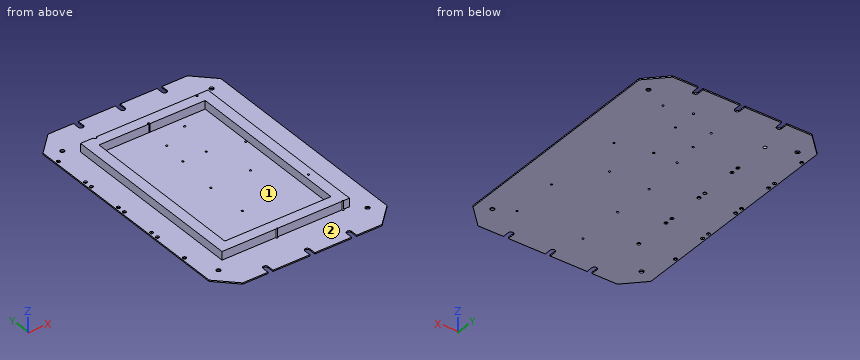
from build123d import *

# Parameters (mm, degrees)
BOSS_EXTRUDE1_DEPTH      = 0.75
BOSS_EXTRUDE1_DEPTH_BACK = 0.75
CUT_EXTRUDE1_DEPTH       = 190.772483022
LPATTERN1_COUNT          = 7
LPATTERN1_PITCH          = 50
MIRROR1_COPY_1_DEPTH     = 190.772483022
MIRROR1_COPY_2_DEPTH     = 190.772483022
MIRROR1_COPY_3_DEPTH     = 190.772483022
MIRROR1_COPY_4_DEPTH     = 190.772483022
MIRROR1_COPY_5_DEPTH     = 190.772483022
MIRROR1_COPY_6_DEPTH     = 190.772483022
SKETCH6_W                = 152.4
SKETCH6_H                = 228.6
SKETCH6_W_2              = 127
SKETCH6_H_2              = 203.2
BOSS_EXTRUDE2_DEPTH      = 11.5
SKETCH7_R                = 2.54
CUT_EXTRUDE2_DEPTH       = 191.11912795
CUT_EXTRUDE3_DEPTH       = 191.11912795
CUT_EXTRUDE3_DEPTH_BACK  = 191.11912795
SKETCH8_R                = 1.15
CUT_EXTRUDE4_DEPTH       = 191.11912795


with BuildPart() as part:
    # Sketch3 → Boss-Extrude1 (new, two sides: drawn at the far end of the back side and taken through both)
    with BuildSketch(Plane.XY.offset(-BOSS_EXTRUDE1_DEPTH_BACK)):
        Polygon((-106.3625, 134.1625), (-83.3625, 157.1625), (83.3625, 157.1625), (106.3625, 134.1625), (106.3625, -134.1625), (83.3625, -157.1625), (-83.3625, -157.1625), (-106.3625, -134.1625), align=None)
    extrude(amount=BOSS_EXTRUDE1_DEPTH + BOSS_EXTRUDE1_DEPTH_BACK)

    # Sketch4 → Cut-Extrude1 (cut, symmetric)
    with BuildSketch(Plane.XY):
        with BuildLine():
            Line((53, 149.225), (53, 157.1625))
            Line((53, 157.1625), (47, 157.1625))
            Line((47, 157.1625), (47, 149.225))
            ThreePointArc((47, 149.225), (50, 146.225), (53, 149.225))
        make_face()
    cut_extrude1 = extrude(amount=CUT_EXTRUDE1_DEPTH, both=True, mode=Mode.SUBTRACT)

    # LPattern1: Cut-Extrude1 ×7
    with Locations(*[(-i * LPATTERN1_PITCH, 0, 0) for i in range(1, LPATTERN1_COUNT)]):
        add(cut_extrude1, mode=Mode.SUBTRACT)

    # Mirror1: Cut-Extrude1 across plane
    add(cut_extrude1.mirror(Plane.ZX), mode=Mode.SUBTRACT)

    # Mirror1 copy 1 sketch → Mirror1 copy 1 (cut, symmetric)
    with BuildSketch(Plane(origin=(-50, 0, 0), x_dir=(1, 0, 0), z_dir=(0, 0, 1))):
        with BuildLine():
            Line((53, -149.225), (53, -157.1625))
            Line((53, -157.1625), (47, -157.1625))
            Line((47, -157.1625), (47, -149.225))
            ThreePointArc((47, -149.225), (50, -146.225), (53, -149.225))
        make_face()
    extrude(amount=MIRROR1_COPY_1_DEPTH, both=True, mode=Mode.SUBTRACT)

    # Mirror1 copy 2 sketch → Mirror1 copy 2 (cut, symmetric)
    with BuildSketch(Plane(origin=(-100, 0, 0), x_dir=(1, 0, 0), z_dir=(0, 0, 1))):
        with BuildLine():
            Line((53, -149.225), (53, -157.1625))
            Line((53, -157.1625), (47, -157.1625))
            Line((47, -157.1625), (47, -149.225))
            ThreePointArc((47, -149.225), (50, -146.225), (53, -149.225))
        make_face()
    extrude(amount=MIRROR1_COPY_2_DEPTH, both=True, mode=Mode.SUBTRACT)

    # Mirror1 copy 3 sketch → Mirror1 copy 3 (cut, symmetric)
    with BuildSketch(Plane(origin=(-150, 0, 0), x_dir=(1, 0, 0), z_dir=(0, 0, 1))):
        with BuildLine():
            Line((53, -149.225), (53, -157.1625))
            Line((53, -157.1625), (47, -157.1625))
            Line((47, -157.1625), (47, -149.225))
            ThreePointArc((47, -149.225), (50, -146.225), (53, -149.225))
        make_face()
    extrude(amount=MIRROR1_COPY_3_DEPTH, both=True, mode=Mode.SUBTRACT)

    # Mirror1 copy 4 sketch → Mirror1 copy 4 (cut, symmetric)
    with BuildSketch(Plane(origin=(-200, 0, 0), x_dir=(1, 0, 0), z_dir=(0, 0, 1))):
        with BuildLine():
            Line((53, -149.225), (53, -157.1625))
            Line((53, -157.1625), (47, -157.1625))
            Line((47, -157.1625), (47, -149.225))
            ThreePointArc((47, -149.225), (50, -146.225), (53, -149.225))
        make_face()
    extrude(amount=MIRROR1_COPY_4_DEPTH, both=True, mode=Mode.SUBTRACT)

    # Mirror1 copy 5 sketch → Mirror1 copy 5 (cut, symmetric)
    with BuildSketch(Plane(origin=(-250, 0, 0), x_dir=(1, 0, 0), z_dir=(0, 0, 1))):
        with BuildLine():
            Line((53, -149.225), (53, -157.1625))
            Line((53, -157.1625), (47, -157.1625))
            Line((47, -157.1625), (47, -149.225))
            ThreePointArc((47, -149.225), (50, -146.225), (53, -149.225))
        make_face()
    extrude(amount=MIRROR1_COPY_5_DEPTH, both=True, mode=Mode.SUBTRACT)

    # Mirror1 copy 6 sketch → Mirror1 copy 6 (cut, symmetric)
    with BuildSketch(Plane(origin=(-300, 0, 0), x_dir=(1, 0, 0), z_dir=(0, 0, 1))):
        with BuildLine():
            Line((53, -149.225), (53, -157.1625))
            Line((53, -157.1625), (47, -157.1625))
            Line((47, -157.1625), (47, -149.225))
            ThreePointArc((47, -149.225), (50, -146.225), (53, -149.225))
        make_face()
    extrude(amount=MIRROR1_COPY_6_DEPTH, both=True, mode=Mode.SUBTRACT)

    # Sketch6 → Boss-Extrude2 (add)
    with BuildSketch(Plane(origin=(0, 0, -0.75), x_dir=(-1, 0, 0), z_dir=(0, 0, -1))):
        Rectangle(SKETCH6_W, SKETCH6_H)
        Rectangle(SKETCH6_W_2, SKETCH6_H_2, mode=Mode.SUBTRACT)
    extrude(amount=-BOSS_EXTRUDE2_DEPTH)

    # Sketch7 → Cut-Extrude2 (cut, through all)
    with BuildSketch(Plane(origin=(0, 0, -0.75), x_dir=(-1, 0, 0), z_dir=(0, 0, -1))):
        with Locations((89.2175, 126.0475)):
            Circle(SKETCH7_R)
        with Locations((-89.2175, 126.0475)):
            Circle(SKETCH7_R)
        with Locations((-89.2175, -126.0475)):
            Circle(SKETCH7_R)
        with Locations((89.2175, -126.0475)):
            Circle(SKETCH7_R)
    extrude(amount=-CUT_EXTRUDE2_DEPTH, mode=Mode.SUBTRACT)

    # Sketch8 → Cut-Extrude3 (cut, two sides: drawn at the far end of the back side and taken through both)
    with BuildSketch(Plane(origin=(0, 0, -0.75), x_dir=(-1, 0, 0), z_dir=(0, 0, -1)).offset(-CUT_EXTRUDE3_DEPTH_BACK)):
        with Locations((-30.1625, 119.0625)):
            Circle(SKETCH8_R)
        with Locations((3.3375, 102.5625)):
            Circle(SKETCH8_R)
        with Locations((-30.1625, 89.8625)):
            Circle(SKETCH8_R)
        with Locations((3.3375, 73.3625)):
            Circle(SKETCH8_R)
        with Locations((-21.2725, 42.8625)):
            Circle(SKETCH8_R)
        with Locations((6.6675, 42.8625)):
            Circle(SKETCH8_R)
        with Locations((-36.5125, -7.9375)):
            Circle(SKETCH8_R)
        with Locations((11.7475, -9.2075)):
            Circle(SKETCH8_R)
        with Locations((-68.2625, -58.7375)):
            Circle(SKETCH8_R)
        with Locations((10.7375, -58.7375)):
            Circle(SKETCH8_R)
        with Locations((10.7375, -114.7375)):
            Circle(SKETCH8_R)
        with Locations((-68.2625, -114.7375)):
            Circle(SKETCH8_R)
        with Locations((-61.9125, 112.7125)):
            Circle(SKETCH8_R)
        with Locations((-61.9125, 33.7125)):
            Circle(SKETCH8_R)
    extrude(amount=CUT_EXTRUDE3_DEPTH + CUT_EXTRUDE3_DEPTH_BACK, mode=Mode.SUBTRACT)

    # Sketch10 → Cut-Extrude4 (cut, through all)
    with BuildSketch(Plane(origin=(0, 0, -0.75), x_dir=(-1, 0, 0), z_dir=(0, 0, -1))):
        with BuildLine():
            ThreePointArc((59.0677, -91.718), (61.0489, -89.7368), (59.0677, -87.7556))
            ThreePointArc((59.0677, -87.7556), (57.0865, -89.7368), (59.0677, -91.718))
        make_face()
        with BuildLine():
            ThreePointArc((59.0677, -38.378), (61.0489, -36.3968), (59.0677, -34.4156))
            ThreePointArc((59.0677, -34.4156), (57.0865, -36.3968), (59.0677, -38.378))
        make_face()
        with BuildLine():
            ThreePointArc((59.0677, -47.903), (61.0489, -45.9218), (59.0677, -43.9406))
            ThreePointArc((59.0677, -43.9406), (57.0865, -45.9218), (59.0677, -47.903))
        make_face()
        with BuildLine():
            ThreePointArc((59.0677, 5.437), (61.0489, 7.4182), (59.0677, 9.3994))
            ThreePointArc((59.0677, 9.3994), (57.0865, 7.4182), (59.0677, 5.437))
        make_face()
        with BuildLine():
            ThreePointArc((59.0677, 14.962), (61.0489, 16.9432), (59.0677, 18.9244))
            ThreePointArc((59.0677, 18.9244), (57.0865, 16.9432), (59.0677, 14.962))
        make_face()
        with BuildLine():
            ThreePointArc((59.0677, 58.777), (61.0489, 60.7582), (59.0677, 62.7394))
            ThreePointArc((59.0677, 62.7394), (57.0865, 60.7582), (59.0677, 58.777))
        make_face()
        with BuildLine():
            ThreePointArc((59.0677, 68.302), (61.0489, 70.2832), (59.0677, 72.2644))
            ThreePointArc((59.0677, 72.2644), (57.0865, 70.2832), (59.0677, 68.302))
        make_face()
        with BuildLine():
            ThreePointArc((59.0677, 112.117), (61.0489, 114.0982), (59.0677, 116.0794))
            ThreePointArc((59.0677, 116.0794), (57.0865, 114.0982), (59.0677, 112.117))
        make_face()
        with BuildLine():
            ThreePointArc((102.8827, 68.302), (104.8639, 70.2832), (102.8827, 72.2644))
            ThreePointArc((102.8827, 72.2644), (100.9015, 70.2832), (102.8827, 68.302))
        make_face()
        with BuildLine():
            ThreePointArc((102.8827, 112.117), (104.8639, 114.0982), (102.8827, 116.0794))
            ThreePointArc((102.8827, 116.0794), (100.9015, 114.0982), (102.8827, 112.117))
        make_face()
        with BuildLine():
            ThreePointArc((102.8827, 14.962), (104.8639, 16.9432), (102.8827, 18.9244))
            ThreePointArc((102.8827, 18.9244), (100.9015, 16.9432), (102.8827, 14.962))
        make_face()
        with BuildLine():
            ThreePointArc((102.8827, 58.777), (104.8639, 60.7582), (102.8827, 62.7394))
            ThreePointArc((102.8827, 62.7394), (100.9015, 60.7582), (102.8827, 58.777))
        make_face()
        with BuildLine():
            ThreePointArc((102.8827, -38.378), (104.8639, -36.3968), (102.8827, -34.4156))
            ThreePointArc((102.8827, -34.4156), (100.9015, -36.3968), (102.8827, -38.378))
        make_face()
        with BuildLine():
            ThreePointArc((102.8827, 5.437), (104.8639, 7.4182), (102.8827, 9.3994))
            ThreePointArc((102.8827, 9.3994), (100.9015, 7.4182), (102.8827, 5.437))
        make_face()
        with BuildLine():
            ThreePointArc((102.8827, -47.903), (104.8639, -45.9218), (102.8827, -43.9406))
            ThreePointArc((102.8827, -43.9406), (100.9015, -45.9218), (102.8827, -47.903))
        make_face()
        with BuildLine():
            ThreePointArc((102.8827, -91.718), (104.8639, -89.7368), (102.8827, -87.7556))
            ThreePointArc((102.8827, -87.7556), (100.9015, -89.7368), (102.8827, -91.718))
        make_face()
    extrude(amount=-CUT_EXTRUDE4_DEPTH, mode=Mode.SUBTRACT)


solid = part.part
Verification items for the finished model (mm, model axes). Face numbers are marked on the shaded views. Give positions to 0.01 mm unless a question says otherwise; leave off trailing zeros. Write each loop counter-clockwise with the first axis right and the second up, starting at its lowest first coordinate (ties: lowest second). Pieces come first, ordered by that corner, then holes. Notation, with made-up numbers: M 80,25.25 L 127,25.25 A22 ccw 127,51.25 Z; hole C 69.5,2.25 d9. An arc over 180 degrees is marked long. Put each result on its own line as item: value. Start each with the question number.
1. Scan lines: line 1 along X through (y, z) = (60, 2.25); line 2 along Y through (x, z) = (12, 5); line 3 along Z through (x, y) = (-4, -3). Record each from-to range of solid material in increasing order. Write a range as [from, to].
2. Section check A-A (x = 41). Record the cut outline in (y, z), and give its area (3 significant figures).
3. Section check C-C (y = -18.5). Record the cut outline in (x, z), and give its area (3 significant figures).
4. Draft check along Y on the marked faces 1 and 2. Enter one of: +Y half, -Y half, draft (parallel to the pull), parting line (faces both ways), or undercut.
5. Go/stop test with flat-tipped pins: pin 1 Ø1.2 at (y, z) = (-153.5, 0) entering from +X (3 decimals); pin 2 Ø1.5 at (x, z) = (-10, 3.5) entering from -Y; pin 3 Ø3 at (x, y) = (-6.67, 42.86) entering from +Z; pin 4 Ø3.5 at (x, y) = (68.26, -58.74) entering from -Z. Record where each tip stops, or that it passes through.
6. Section check B-B (z = 2.75). Record the cut outline in (x, y).
Answer list:
1. line 1: [-76.2, -63.5], [63.5, 76.2]
1. line 2: [-114.3, -101.6], [101.6, 114.3]
1. line 3: [-0.75, 0.75]
2. outline: M -157.16,-0.75 L 157.16,-0.75 L 157.16,0.75 L 114.3,0.75 L 114.3,10.75 L 101.6,10.75 L 101.6,0.75 L -101.6,0.75 L -101.6,10.75 L -114.3,10.75 L -114.3,0.75 L -157.16,0.75 Z
2. area: 725 mm2
3. outline: M -106.36,-0.75 L 106.36,-0.75 L 106.36,0.75 L 76.2,0.75 L 76.2,10.75 L 63.5,10.75 L 63.5,0.75 L -63.5,0.75 L -63.5,10.75 L -76.2,10.75 L -76.2,0.75 L -106.36,0.75 Z
3. area: 573 mm2
4. face 1: undercut
4. face 2: draft
5. pin 1: x = 87.625
5. pin 2: y = -114.3
5. pin 3: z = 0.75
5. pin 4: z = -0.75
6. outline: M -76.2,-114.3 L -11.8,-114.3 A1.15 cw -9.67,-114.3 L 67.2,-114.3 A1.15 cw 69.33,-114.3 L 76.2,-114.3 L 76.2,114.3 L -57.1,114.3 A1.98 cw long -61.04,114.3 L -76.2,114.3 Z; hole M -63.5,-101.6 L 63.5,-101.6 L 63.5,101.6 L -2.71,101.6 A1.15 ccw long -3.97,101.6 L -63.5,101.6 Z; hole C 61.91,112.71 d2.3; hole C 68.26,-58.74 d2.3
